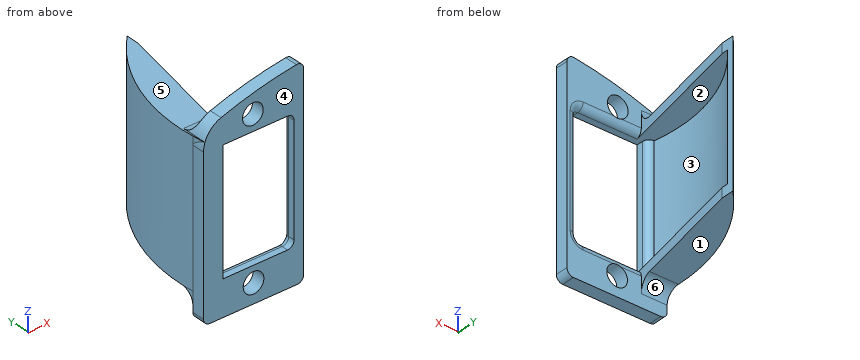
```python
from build123d import *

# Parameters (mm, degrees)
SKETCH1_W                = 11
SKETCH1_H                = 19
BOSS_EXTRUDE1_DEPTH      = 2
BOSS_EXTRUDE2_DEPTH      = 11
BOSS_EXTRUDE2_DEPTH_BACK = 11
BOSS_EXTRUDE3_DEPTH      = 1.5
BOSS_EXTRUDE4_START      = -22
BOSS_EXTRUDE4_DEPTH      = 1.5
SKETCH4_R                = 1.6
CUT_EXTRUDE1_DEPTH       = 41.722097522
FILLET1_R                = 4
FILLET2_R                = 1
FILLET3_R                = 2


with BuildPart() as part:
    # Sketch1 → Boss-Extrude1 (new body)
    with BuildSketch(Plane(origin=(0, 0, 0), x_dir=(1, 0, 0), z_dir=(0, 1, 0))):
        with BuildLine():
            Line((-0.004910497, 3.064545275), (-0.004910497, 30.564545275))
            Line((-0.004910497, 30.564545275), (15.495089503, 30.564545275))
            Line((15.495089503, 30.564545275), (15.495089503, -0.81352161))
            ThreePointArc((15.495089503, -0.81352161), (7.615422876, 0.607255499), (-0.004910497, 3.064545275))
        make_face()
        with Locations((8.495089503, 15.564545275)):
            Rectangle(SKETCH1_W, SKETCH1_H, mode=Mode.SUBTRACT)
    extrude(amount=BOSS_EXTRUDE1_DEPTH)

    # Sketch2 → Boss-Extrude2 (add, two sides: drawn at the far end of the back side and taken through both)
    with BuildSketch(Plane.XY.offset(-15.564545275).offset(-BOSS_EXTRUDE2_DEPTH_BACK)):
        with BuildLine():
            Line((7.995089503, 24), (7.995089503, 23))
            ThreePointArc((7.995089503, 23), (2.580593395, 13.189856031), (1.995089503, 2))
            Line((1.995089503, 2), (-0.004910497, 2))
            ThreePointArc((-0.004910497, 2), (1.585642128, 13.876162682), (7.995089503, 24))
        make_face()
    extrude(amount=BOSS_EXTRUDE2_DEPTH + BOSS_EXTRUDE2_DEPTH_BACK)

    # Sketch3 → Boss-Extrude3 (add)
    with BuildSketch(Plane.XY.offset(-4.564545275)):
        with BuildLine():
            Line((7.995089503, 24), (7.995089503, 22))
            Line((7.995089503, 22), (3.995089503, 2))
            Line((3.995089503, 2), (-0.004910497, 2))
            ThreePointArc((-0.004910497, 2), (1.760688004, 13.812509636), (7.995089503, 24))
        make_face()
    extrude(amount=-BOSS_EXTRUDE3_DEPTH)

    # Sketch3<2> → Boss-Extrude4 (add)
    with BuildSketch(Plane.XY.offset(-4.564545275).offset(BOSS_EXTRUDE4_START)):
        with BuildLine():
            Line((7.995089503, 24), (7.995089503, 22))
            Line((7.995089503, 22), (3.995089503, 2))
            Line((3.995089503, 2), (-0.004910497, 2))
            ThreePointArc((-0.004910497, 2), (1.760688004, 13.812509636), (7.995089503, 24))
        make_face()
    extrude(amount=BOSS_EXTRUDE4_DEPTH)

    # Sketch4 → Cut-Extrude1 (cut, through all)
    with BuildSketch(Plane(origin=(0, 2, 0), x_dir=(1, 0, 0), z_dir=(0, 1, 0))):
        with Locations(Location((7.732104354, 27.564545275, 0), (0, 0, 270))):
            Circle(SKETCH4_R)
        with Locations(Location((7.628223159, 3.564545275, 0), (0, 0, 270))):
            Circle(SKETCH4_R)
    extrude(amount=-CUT_EXTRUDE1_DEPTH, mode=Mode.SUBTRACT)

    # Fillet1
    # the kernel refuses this fillet: 4 mm, written as the material it takes off along each edge
    with BuildSketch(Plane(origin=(-0.004910497, -7.201261458, -3.064545275), x_dir=(0, 0, -1), z_dir=(0, 1, 0))) as fillet1_piece_1_section:
        with BuildLine():
            CenterArc((2.782831809, -4), FILLET1_R, 90, 71.052480457)
            ThreePointArc((-1.000433732, -2.701192145), (-0.516429194, -1.344591553), (0, 0))
            Line((0, 0), (2.782831809, 0))
        make_face()
    fillet1_piece_1 = extrude(amount=16.402522916, mode=Mode.PRIVATE)
    fillet1_piece_1 = fillet1_piece_1 - Plane(origin=(27.899857986, 4.307356915, -4.929207358), x_dir=(-0.9965988743768334, -0.08240560412271017, 0), z_dir=(0, 0, -1)) * Cylinder(28, 44, mode=Mode.PRIVATE)
    add(fillet1_piece_1, mode=Mode.SUBTRACT)
    with BuildSketch(Plane(origin=(-0.004910497, -7.201261458, -3.064545275), x_dir=(0, 0, -1), z_dir=(0, 1, 0))) as fillet1_piece_2_section:
        with BuildLine():
            CenterArc((2.782831809, -4), FILLET1_R, 90, 71.052480457)
            ThreePointArc((-1.000433732, -2.701192145), (-0.516429194, -1.344591553), (0, 0))
            Line((0, 0), (2.782831809, 0))
        make_face()
    fillet1_piece_2 = extrude(amount=16.402522916, mode=Mode.PRIVATE)
    fillet1_piece_2 = split(fillet1_piece_2, bisect_by=Plane(origin=(0.675993318, 1.051688324, -4.564545275), z_dir=(0, 0, 1)), keep=Keep.TOP, mode=Mode.PRIVATE)
    add(fillet1_piece_2, mode=Mode.SUBTRACT)

    # Fillet2
    # the kernel refuses this fillet: 1 mm, written as the material it adds along each edge
    with BuildSketch(Plane(origin=(13.995089503, 0, -6.064545275), x_dir=(0, 0, -1), z_dir=(0, 1, 0)), Plane(origin=(13.995089503, 0, -25.064545275), x_dir=(-1, 0, 0), z_dir=(0, 1, 0))) as fillet2_piece_1:
        with BuildLine():
            CenterArc((FILLET2_R, FILLET2_R), FILLET2_R, 180, 90)
            Line((0, FILLET2_R), (0, 0))
            Line((0, 0), (FILLET2_R, 0))
        make_face()
    extrude(amount=2)
    # the kernel refuses this fillet: 1 mm, written as the material it takes off along each edge
    with BuildSketch(Plane(origin=(2.995089503, 2, -6.064545275), x_dir=(0, -1, 0), z_dir=(0, 0, -1))) as fillet2_2_piece_1:
        with BuildLine():
            CenterArc((FILLET2_R, FILLET2_R), FILLET2_R, 180, 90)
            Line((0, FILLET2_R), (0, 0))
            Line((0, 0), (FILLET2_R, 0))
        make_face()
    extrude(amount=19, mode=Mode.SUBTRACT)
    with BuildSketch(Plane(origin=(-0.004910497, -2.5, -30.564545275), x_dir=(0, 0, 1), z_dir=(0, 1, 0)), Plane(origin=(15.495089503, -2.5, -30.564545275), x_dir=(-1, 0, 0), z_dir=(0, 1, 0))) as fillet2_2_piece_2:
        with BuildLine():
            CenterArc((FILLET2_R, FILLET2_R), FILLET2_R, 180, 90)
            Line((0, FILLET2_R), (0, 0))
            Line((0, 0), (FILLET2_R, 0))
        make_face()
    extrude(amount=7, mode=Mode.SUBTRACT)
    with BuildSketch(Plane(origin=(15.495089503, -2.846412971, 0.81352161), x_dir=(0, 0, -1), z_dir=(0, 1, 0))) as fillet2_2_piece_3:
        with BuildLine():
            CenterArc((1.129037279, 1), FILLET2_R, 172.517371348, 97.482628652)
            ThreePointArc((0.137552889, 1.130225593), (0.066095477, 0.565439081), (0, 0))
            Line((0, 0), (1.129037279, 0))
        make_face()
    extrude(amount=7.692825941, mode=Mode.SUBTRACT)
    # the kernel refuses this fillet: 1 mm, written as the material it takes off along each edge
    with BuildSketch(Plane(origin=(12.995089503, 2, -6.064545275), x_dir=(0, 0, 1), z_dir=(-1, 0, 0))) as fillet2_3_piece_1_section:
        with BuildLine():
            CenterArc((FILLET2_R, -FILLET2_R), FILLET2_R, 90, 90)
            Line((0, -FILLET2_R), (0, 0))
            Line((0, 0), (FILLET2_R, 0))
        make_face()
    fillet2_3_piece_1 = extrude(amount=11.5, mode=Mode.PRIVATE)
    fillet2_3_piece_1 = split(fillet2_3_piece_1, bisect_by=Plane(origin=(4.123556577, 2.642335372, -5.838757255), z_dir=(0.9805806756909202, -0.19611613513818374, 0)), keep=Keep.TOP, mode=Mode.PRIVATE)
    add(fillet2_3_piece_1, mode=Mode.SUBTRACT)
    with BuildSketch(Plane(origin=(1.495089503, 2, -25.064545275), x_dir=(0, 0, -1), z_dir=(1, 0, 0))) as fillet2_3_piece_2_section:
        with BuildLine():
            CenterArc((FILLET2_R, -FILLET2_R), FILLET2_R, 90, 90)
            Line((0, -FILLET2_R), (0, 0))
            Line((0, 0), (FILLET2_R, 0))
        make_face()
    fillet2_3_piece_2 = extrude(amount=11.5, mode=Mode.PRIVATE)
    fillet2_3_piece_2 = split(fillet2_3_piece_2, bisect_by=Plane(origin=(4.123556577, 2.642335372, -25.290333294), z_dir=(0.9805806756909202, -0.19611613513818374, 0)), keep=Keep.TOP, mode=Mode.PRIVATE)
    add(fillet2_3_piece_2, mode=Mode.SUBTRACT)
    with BuildSketch(Plane(origin=(13.995089503, 2, -24.064545275), x_dir=(1, 0, 0), z_dir=(0, 0, 1))) as fillet2_3_piece_3:
        with BuildLine():
            CenterArc((FILLET2_R, -FILLET2_R), FILLET2_R, 90, 90)
            Line((0, -FILLET2_R), (0, 0))
            Line((0, 0), (FILLET2_R, 0))
        make_face()
    extrude(amount=17, mode=Mode.SUBTRACT)
    with BuildSketch(Plane(origin=(12.995089503, 2, -24.064545275), x_dir=(0, 0, -1), z_dir=(-1, 0, 0))) as fillet2_3_piece_4:
        with BuildLine():
            CenterArc((1 + FILLET2_R, FILLET2_R), FILLET2_R, 180, 90)
            Line((1, FILLET2_R), (1, 0))
            Line((1, 0), (1 + FILLET2_R, 0))
        make_face()
    revolve(axis=Axis((12.995089503, 2, -24.064545275), (0, -1, 0)), revolution_arc=90, mode=Mode.SUBTRACT)
    with BuildSketch(Plane(origin=(12.995089503, 2, -7.064545275), x_dir=(1, 0, 0), z_dir=(0, 0, -1))) as fillet2_3_piece_5:
        with BuildLine():
            CenterArc((1 + FILLET2_R, FILLET2_R), FILLET2_R, 180, 90)
            Line((1, FILLET2_R), (1, 0))
            Line((1, 0), (1 + FILLET2_R, 0))
        make_face()
    revolve(axis=Axis((12.995089503, 2, -7.064545275), (0, -1, 0)), revolution_arc=90, mode=Mode.SUBTRACT)

    # Fillet3
    # the kernel refuses this fillet: 2 mm, written as the material it adds along each edge
    with BuildSketch(Plane(origin=(8.995089503, 2, -4.564545275), x_dir=(0, 0, 1), z_dir=(-1, 0, 0))) as fillet3_piece_1_section:
        with BuildLine():
            CenterArc((FILLET3_R, FILLET3_R), FILLET3_R, 180, 90)
            Line((0, FILLET3_R), (0, 0))
            Line((0, 0), (FILLET3_R, 0))
        make_face()
    fillet3_piece_1 = extrude(amount=13.788712519, mode=Mode.PRIVATE)
    fillet3_piece_1 = fillet3_piece_1 & Plane(origin=(3.995089503, 2.466350157, -5.847377084), x_dir=(0, 0, -1), z_dir=(0, -1, 0)) * Cylinder(4, 36, mode=Mode.PRIVATE)
    fillet3_piece_1 = split(fillet3_piece_1, bisect_by=Plane(origin=(4.017419709, 2.111651029, -4.143772398), z_dir=(-0.9805806756909202, 0.19611613513818374, 0)), keep=Keep.TOP, mode=Mode.PRIVATE)
    add(fillet3_piece_1)
    with BuildSketch(Plane(origin=(-5.004910497, 2, -26.564545275), x_dir=(0, 0, -1), z_dir=(1, 0, 0))) as fillet3_piece_2_section:
        with BuildLine():
            CenterArc((FILLET3_R, FILLET3_R), FILLET3_R, 180, 90)
            Line((0, FILLET3_R), (0, 0))
            Line((0, 0), (FILLET3_R, 0))
        make_face()
    fillet3_piece_2 = extrude(amount=14, mode=Mode.PRIVATE)
    fillet3_piece_2 = fillet3_piece_2 & Plane(origin=(27.899857986, 4.307356915, -26.843512553), x_dir=(-0.9965988743768334, -0.08240560412271017, 0), z_dir=(0, 0, -1)) * Cylinder(28, 36, mode=Mode.PRIVATE)
    fillet3_piece_2 = split(fillet3_piece_2, bisect_by=Plane(origin=(3.978687185, 1.91798841, -26.843512553), z_dir=(-0.9805806756909202, 0.19611613513818374, 0)), keep=Keep.TOP, mode=Mode.PRIVATE)
    add(fillet3_piece_2)


solid = part.part
```
Geometry: final body of the model. Coordinates: model frame, mm. Face numbers are marked on the shaded views. A direction names the side the tool comes from. Round coordinates to 2 decimals unless told otherwise and drop trailing zeros. Loops run counter-clockwise (first coordinate to the right, second up) from the corner with the lowest first, then second, coordinate; pieces in that order, holes last. Notation, with made-up numbers: (-17, -16.5) -> (2, -16.5) arc R27 ccw to (2, 22.5) -> close; hole circle Ø5 at (31, 66.25). An arc over 180 degrees is marked (long way). Write each question's results on one line, items separated by ' | '.
Item 1: Cut plane B-B on y = 8.25. Return the cut outline in (x, z).
Answers below:
outline: (0.18, -26.56) -> (5.25, -26.56) -> (5.25, -25.06) -> (1.69, -25.06) -> (1.69, -6.06) -> (5.25, -6.06) -> (5.25, -4.56) -> (0.18, -4.56) -> close
Item 2: Cut plane A-A on z = -8.5. Return the cut outline in (x, y), and give its area (3 significant figures).
Answers below:
outline: (0, 0) -> (3, 0) -> (3, 1) arc R1 ccw to (2, 2) arc R25 cw to (8, 23) -> (8, 24) arc R28 ccw to (0, 2) -> close; (14, 0) -> (15.5, 0) -> (15.5, 2) -> (15, 2) arc R1 ccw to (14, 1) -> close | area: 37.0 mm²
Item 3: Cut plane D-D on y = 18.25. Return the cut outline in (x, z), and give its area (3 significant figures).
Answers below:
outline: (3.62, -26.56) -> (7.25, -26.56) -> (7.25, -25.06) -> (4.65, -25.06) -> (4.65, -6.06) -> (7.25, -6.06) -> (7.25, -4.56) -> (3.62, -4.56) -> close | area: 30.4 mm²
Item 4: Set-up query: the marked faces 1 and 2. Return all of +Z, -Z, +X, -X, +Y, -Y with unobstructed straight access to the full face (end or side cutting, diameter ignored); none if empty.
Answers below:
face 1: -Z, +X, -X, +Y | face 2: none
Item 5: Pull-direction query (Y, two-part tool) for the marked faces 3, 4, 5 and 6; classes: pulls with the +Y half, pulls with the -Y half, needs draft (parallel to the pull), parting line crosses it, or undercut.
Answers below:
face 3: undercut | face 4: pulls with the -Y half | face 5: needs draft | face 6: pulls with the +Y half
Item 6: Cut plane C-C on x = 11.25. Return the cut outline in (y, z), and give its area (3 significant figures).
Answers below:
outline: (0, -30.56) -> (2, -30.56) -> (2, -26.06) arc R1 ccw to (1, -25.06) -> (0, -25.06) -> close; (0, -6.06) -> (1, -6.06) arc R1 ccw to (2, -5.06) -> (2, 0.18) -> (0, 0.18) -> close | area: 23.1 mm²
Item 7: Line query: probe 1 along Z at (x, y) = (2.25, 5.75); probe 2 along Z at (x, y) = (1.5, 8); probe 3 along Y at (x, z) = (9, -2.5). Output: solid intervals per line, ascending. Write a range as [from, to].
Answers below:
probe 1: z = [-26.56, -25.06], [-6.06, -4.56] | probe 2: z = [-26.56, -4.56] | probe 3: y = [0, 2]
Item 8: Pin query (flat end, axial travel): pin 1 Ø6 at (x, z) = (12, -7.5) entering from -Y; pin 2 Ø2 at (y, z) = (0.5, -18.5) entering from -X; pin 3 Ø1.5 at (y, z) = (18, -16.5) entering from -X; pin 4 Ø5 at (x, y) = (12, 21.5) entering from -Z. Return the tip coordinate at first contact, or that it passes through.
Answers below:
pin 1: stops at y = 0 | pin 2: stops at x = 0 | pin 3: stops at x = 3.07 | pin 4: passes through
